```python
from build123d import *

# Parameters (mm, degrees)
F0_W     = 50.8
F0_H     = 101.6
F1_DEPTH = 50.8
F3_DEPTH = 50.8
F5_DEPTH = 50.8


with BuildPart() as f1:
    # F0 (on Right) → F1 (new body)
    with BuildSketch(Plane.YZ):
        Polygon((0, 86.36), (-25.4, 50.8), (25.4, 50.8), align=None)
        Rectangle(F0_W, F0_H)
        Polygon((25.4, -50.8), (-25.4, -50.8), (0, -86.36), align=None)
    extrude(amount=F1_DEPTH)

    # F2 (on face) → F3 (cut)
    with BuildSketch(Plane(origin=(0, 25.4, 0), x_dir=(-1, 0, 0), z_dir=(0, 1, 0))):
        Polygon((-50.8, 86.36), (-50.8, 50.8), (-25.4, 86.36), align=None)
        Polygon((-25.4, 86.36), (0, 50.8), (0, 86.36), align=None)
    extrude(amount=-F3_DEPTH, mode=Mode.SUBTRACT)

    # F4 (on face) → F5 (cut)
    with BuildSketch(Plane(origin=(0, 25.4, 0), x_dir=(-1, 0, 0), z_dir=(0, 1, 0))):
        Polygon((0, -86.36), (0, -50.8), (-25.4, -86.36), align=None)
        Polygon((-25.4, -86.36), (-50.8, -50.8), (-50.8, -86.36), align=None)
    extrude(amount=-F5_DEPTH, mode=Mode.SUBTRACT)


solid = f1.part
```
Geometry check sheet. Reference: the model listing, model coordinates, mm. Round coordinates to 2 decimals unless told otherwise and drop trailing zeros. Order: outer loops, then holes, each group sorted by start corner. A loop starts at its lowest first (then second) coordinate and runs counter-clockwise, first axis right, second up. Notation, with made-up numbers: M 35.5,-3 L 94.5,-3 A8 ccw 94.5,3 Z; hole C 29.5,-12 d8. An arc over 180 degrees is marked long. Write item = value, one per line.
Q1. Section check B-B (y = -6.5). Enter the section's corners in (x, z).
Answer block:
outline = M 0,-50.8 L 18.9,-77.26 L 31.9,-77.26 L 50.8,-50.8 L 50.8,50.8 L 31.9,77.26 L 18.9,77.26 L 0,50.8 Z
Q2. Section check A-A (x = 19.5). Enter the section's corners in (y, z), plus the area to 3 significant figures.
Answer block:
outline = M -25.4,-50.8 L -5.9,-78.1 L 5.9,-78.1 L 25.4,-50.8 L 25.4,50.8 L 5.9,78.1 L -5.9,78.1 L -25.4,50.8 Z
area = 6,870 mm^2
Q3. Scan lines: line 1 (Y direction, x = 14, z = 62); line 2 (Z direction, x = 40, y = -19); line 3 (Y direction, x = 13, z = -67.5). Record each from-to range of solid material in increasing order.
Answer block:
line_1 = -17.4 to 17.4
line_2 = -59.76 to 59.76
line_3 = -13.47 to 13.47
Q4. Section check C-C (z = -59). Enter the section's corners in (x, y), plus the area to 3 significant figures.
Answer block:
outline = M 5.86,-19.54 L 44.94,-19.54 L 44.94,19.54 L 5.86,19.54 Z
area = 1,530 mm^2
Q5. Depth check by flat-ended pin: pin 1 Ø6 at (x, y) = (29, -19.5) entering from +Z; pin 2 Ø10 at (x, y) = (18, -12.5) entering from +Z; pin 3 Ø1.5 at (y, z) = (19, 59.5) entering from +X. Enter the tip coordinate at first touch or a pass-through.
Answer block:
pin_1 = 63.26
pin_2 = 75.86
pin_3 = 45.12
